from build123d import *

# Parameters (mm, degrees)
F1_DEPTH = 25.4


with BuildPart() as f1:
    # F0 (on Top) → F1 (new body)
    with BuildSketch(Plane.XY):
        Polygon((-11.6460118443, 43.6722375453), (20.3620182707, 20.1480132985), (31.6143950059, 31.2821274658), align=None)
        Polygon((75.2486810088, 74.4578167796), (31.6143950059, 31.2821274658), (54.9272783101, 24.60514009), (40.5425727367, 5.3163636476), (1.5286983689, -0.4096143239), (75.2486810088, -76.0029926896), align=None)
        Polygon((31.6143950059, 31.2821274658), (20.3620182707, 20.1480132985), (40.5425727367, 5.3163636476), (54.9272783101, 24.60514009), align=None)
    extrude(amount=-F1_DEPTH)


solid = f1.part
Can you work these out from the model? Positions are in its coordinate system, mm. A direction names the side the tool comes from. Coordinates: 2 decimals unless noted, no trailing zeros. Loops run counter-clockwise (first coordinate to the right, second up) from the corner with the lowest first, then second, coordinate; pieces in that order, holes last. Notation, with made-up numbers: (-27.75, 67) - (17.25, 67) arc R18 cw to (17.25, 85) - close; hole circle Ø2 at (-21, 70). An arc over 180 degrees is marked (long way). Answer as a JSON object with one key per item and string values. Group by question number.
Item 1: If we section it at C-C (x = 15.5): List the corners of the cut face in (y, z) for me, plus the area to 3 significant figures.
Item 2: If we section it at A-A (x = 38): List the corners of the cut face in (y, z) for me.
Item 3: For pin 1 (10 mm diameter, centred on x = 15.5, z = -5.5, fed in from -Y); pin 2 (2 mm diameter, centred on x = 35, z = -13, fed in from +Y); pin 3 (5 mm diameter, centred on y = 47.5, z = -22.5, fed in from -X), each with a flat end and sliding along its axis, tell me the tip position at first contact or that it passes through.
Item 4: On a 3-axis mill with a long thin cutter (end or side, diameter ignored), from which of +Z, -Z, +X, -X, +Y, -Y can I reach the whole of each face in a straight line? I mean faces 1 (the face through (75.249, -2, -13)), 2 (the face through (21.309, 2.493, -12.522)). Say none if no direction works.
Item 5: If we section it at D-D (y = 12.5): List the corners of the cut face in (x, z) for me, plus the area to 3 significant figures.
Item 6: If we section it at B-B (z = -6.5): List the corners of the cut face in (x, y) for me, plus the area to 3 significant figures.
Item 7: If I drill on L1, parallel to Y at x = 26, z = -15.25; L2, parallel to Y at x = 35, z = -17.25; L3, parallel to X at y = 50, z = -6.25, over which ranges is the centre line in solid material (lowest first)? Write a range as from..to.
Item 8: If we mould it in two halves opening along X, with no side actions, what happens to faces 3 (the face through (37.873, -37.677, -12.522)), 4 (the face through (51, 0, -25.4)), 5 (the face through (53.737, 53.172, -12.522)), 6 (the face through (10.29, 37.39, -12.52))? For each: released by +X, released by -X, zero draft, split by the parting line, or undercut.
Returned:
{
 "1": {"outline": "(-14.74, -25.4) - (1.64, -25.4) - (1.64, 0) - (-14.74, 0) - close; (23.72, -25.4) - (35.9, -25.4) - (35.9, 0) - (23.72, 0) - close", "area": "725 mm²"},
 "2": {"outline": "(-37.81, -25.4) - (4.94, -25.4) - (4.94, 0) - (-37.81, 0) - close; (7.19, -25.4) - (37.6, -25.4) - (37.6, 0) - (7.19, 0) - close"},
 "3": {"pin 1": "stops at y = -19.86", "pin 2": "stops at y = 35.62", "pin 3": "stops at x = 45.48"},
 "4": {"face 1": "+Z, -Z, +X, +Y, -Y", "face 2": "+Z, -Z, -X"},
 "5": {"outline": "(30.77, -25.4) - (75.25, -25.4) - (75.25, 0) - (30.77, 0) - close", "area": "1,130 mm²"},
 "6": {"outline": "(-11.65, 43.67) - (40.54, 5.32) - (1.53, -0.41) - (75.25, -76) - (75.25, 74.46) - (31.61, 31.28) - close", "area": "5,560 mm²"},
 "7": {"L1": "y = -25.5..3.18, 16..32.89", "L2": "y = -34.73..4.5, 9.39..34.63", "L3": "x = 50.53..75.25"},
 "8": {"face 3": "released by -X", "face 4": "zero draft", "face 5": "undercut", "face 6": "undercut"}
}
